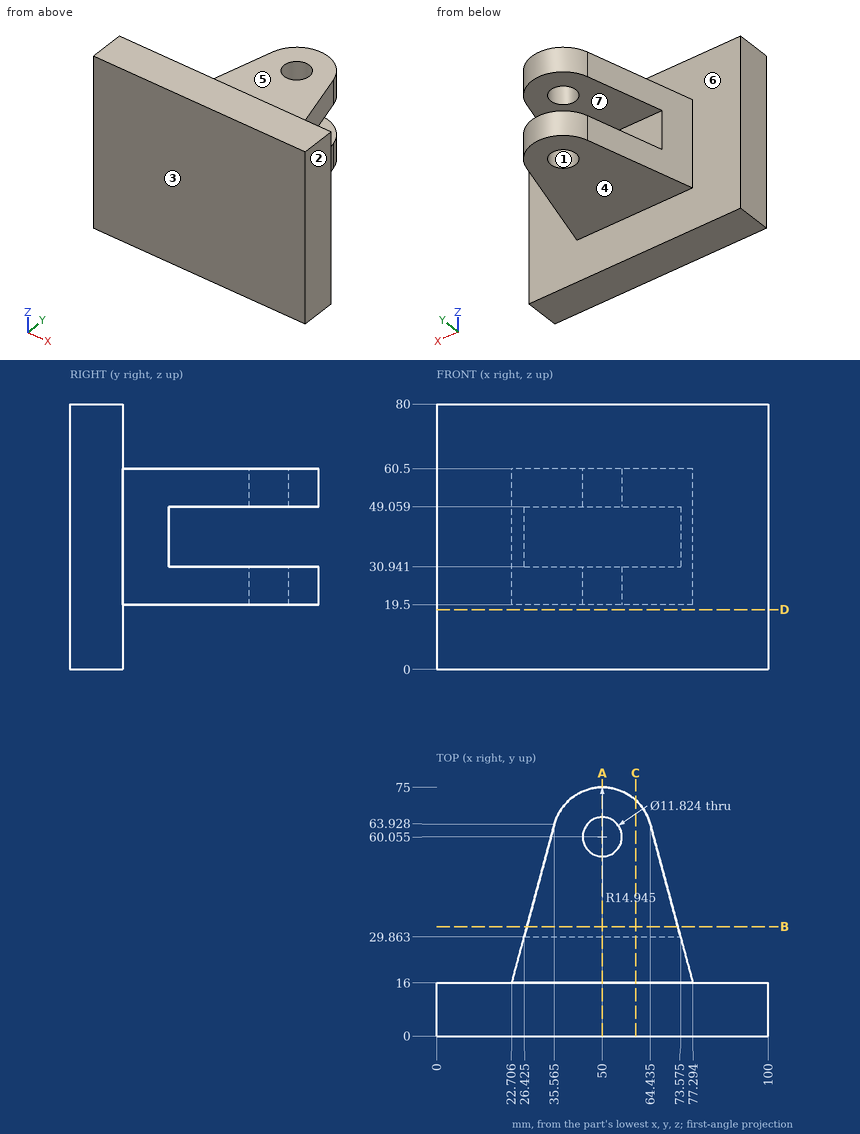
Geometry check sheet. Reference: drawing and pictorial views, mm from the part's lowest x, y, z. A direction names the side the tool comes from. Round coordinates to 2 decimals unless told otherwise and drop trailing zeros. Order: outer loops, then holes, each group sorted by start corner. A loop starts at its lowest first (then second) coordinate and runs counter-clockwise, first axis right, second up. Notation, with made-up numbers: (-24.75, 68.25) - (18.25, 68.25) arc R4 cw to (18.25, 74.25) - close; hole circle Ø5 at (13, 72.5). An arc over 180 degrees is marked (long way). Write item = value, one per line.
Q1. Section check C-C (x = 60). Record the boundary of the cut face in (y, z).
Computed:
outline = (0, 0) - (16, 0) - (16, 19.5) - (71.16, 19.5) - (71.16, 30.94) - (29.86, 30.94) - (29.86, 49.06) - (71.16, 49.06) - (71.16, 60.5) - (16, 60.5) - (16, 80) - (0, 80) - close
Q2. Tool access check on the marked faces 4, 5, 6 and 7. Record the directions out of +Z, -Z, +X, -X, +Y, -Y that give a thin tool (end or side, any length) a straight path to the whole face; none if there is none.
Computed:
face_4 = -Z, +X, -X, +Y
face_5 = +Z, +X, -X, +Y
face_6 = +Y
face_7 = +X, -X, +Y
Q3. Draft check along Y on the marked faces 1, 2 and 3. Enter one of: pulls with the +Y half, pulls with the -Y half, needs draft (parallel to the pull), parting line crosses it, or undercut.
Computed:
face_1 = undercut
face_2 = needs draft
face_3 = pulls with the -Y half
Q4. Section check D-D (z = 18). Record the boundary of the cut face in (x, y).
Computed:
outline = (0, 0) - (100, 0) - (100, 16) - (0, 16) - close
Q5. Section check B-B (y = 33). Record the boundary of the cut face in (x, z), and give its area (3 significant figures).
Computed:
outline = (27.27, 19.5) - (72.73, 19.5) - (72.73, 30.94) - (27.27, 30.94) - close; (27.27, 49.06) - (72.73, 49.06) - (72.73, 60.5) - (27.27, 60.5) - close
area = 1,040 mm^2
Q6. Section check A-A (x = 50). Record the boundary of the cut face in (y, z), and give its area (3 significant figures).
Computed:
outline = (0, 0) - (16, 0) - (16, 19.5) - (54.14, 19.5) - (54.14, 30.94) - (29.86, 30.94) - (29.86, 49.06) - (54.14, 49.06) - (54.14, 60.5) - (16, 60.5) - (16, 80) - (0, 80) - close; (65.97, 19.5) - (75, 19.5) - (75, 30.94) - (65.97, 30.94) - close; (65.97, 49.06) - (75, 49.06) - (75, 60.5) - (65.97, 60.5) - close
area = 2,610 mm^2
Q7. Go/stop test with flat-tipped pins: pin 1 (5 mm diameter, centred on y = 15, z = 65.5, fed in from -X); pin 2 (8 mm diameter, centred on y = 45.5, z = 51, fed in from +X); pin 3 (7 mm diameter, centred on x = 50, y = 60.05, fed in from +Z); pin 4 (12 mm diameter, centred on y = 56.5, z = 27.5, fed in from -X). Record where each tip stops, or that it passes through.
Computed:
pin_1 = 0
pin_2 = 70.45
pin_3 = through
pin_4 = 31.96
Q8. Thickness scan on line 1 along Y through (x, z) = (50, 53); line 2 along Z through (x, y) = (50.5, 33.5); line 3 along Z through (x, y) = (56, 20). Record the ranges inside material, lowest first.
Computed:
line_1 = 0 to 54.14, 65.97 to 75
line_2 = 19.5 to 30.94, 49.06 to 60.5
line_3 = 19.5 to 60.5
